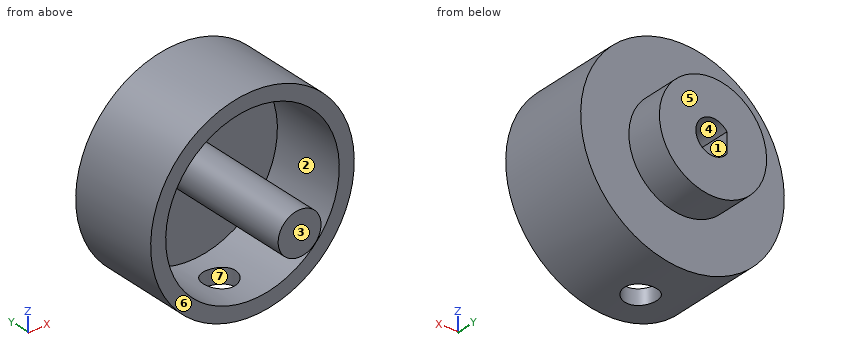
```python
from build123d import *

# Parameters (mm, degrees)
ESQUISSE1_R             = 4
BOSS_EXTRU_1_DEPTH      = 35
ESQUISSE2_R             = 3.2
ENL_V_MAT_EXTRU_1_DEPTH = 13
BOSS_EXTRU_2_START      = 13
BOSS_EXTRU_2_DEPTH      = 13
ESQUISSE5_R             = 10
ESQUISSE5_R_2           = 4
BOSS_EXTRU_3_DEPTH      = 7
SKETCH2_R               = 16.2
SKETCH2_R_2             = 4
BOSS_EXTRUDE4_DEPTH     = 3
SKETCH2_8_R             = 19
SKETCH2_8_R_2           = 16.2
BOSS_EXTRUDE5_DEPTH     = 17.2
SKETCH4_R               = 3
CUT_EXTRUDE1_DEPTH      = 10


with BuildPart() as part:
    # Esquisse1 → Boss.-Extru.1 (new body)
    with BuildSketch(Plane(origin=(0, 0, 0), x_dir=(1, 0, 0), z_dir=(0, 1, 0))):
        with Locations(Location((0, 0, 0), (0, 0, 270))):
            Circle(ESQUISSE1_R)
    extrude(amount=-BOSS_EXTRU_1_DEPTH)

    # Esquisse2 → Enl_v. mat.-Extru.1 (cut)
    with BuildSketch(Plane(origin=(0, 0, 0), x_dir=(1, 0, 0), z_dir=(0, 1, 0))):
        with Locations(Location((0, 0, 0), (0, 0, 270))):
            Circle(ESQUISSE2_R)
    extrude(amount=-ENL_V_MAT_EXTRU_1_DEPTH, mode=Mode.SUBTRACT)

    # Esquisse4 → Boss.-Extru.2 (add)
    with BuildSketch(Plane(origin=(0, -13, 0), x_dir=(1, 0, 0), z_dir=(0, 1, 0)).offset(BOSS_EXTRU_2_START)):
        with BuildLine():
            Line((-2.6, -1.865475811), (-2.6, 0))
            Line((-2.6, 0), (-2.6, 1.865475811))
            ThreePointArc((-2.6, 1.865475811), (-3.2, 0), (-2.6, -1.865475811))
        make_face()
    extrude(amount=-BOSS_EXTRU_2_DEPTH)

    # Esquisse5 → Boss.-Extru.3 (add)
    with BuildSketch(Plane(origin=(0, 0, 0), x_dir=(1, 0, 0), z_dir=(0, 1, 0))):
        with Locations(Location((0, 0, 0), (0, 0, 270))):
            Circle(ESQUISSE5_R)
        with Locations(Location((0, 0, 0), (0, 0, 270))):
            Circle(ESQUISSE5_R_2, mode=Mode.SUBTRACT)
    extrude(amount=-BOSS_EXTRU_3_DEPTH)

    # Sketch2 → Boss-Extrude4 (add)
    with BuildSketch(Plane.XZ.offset(7)):
        with Locations(Location((0, 0, 0), (0, 0, 270))):
            Circle(SKETCH2_R)
        with Locations(Location((0, 0, 0), (0, 0, 90))):
            Circle(SKETCH2_R_2, mode=Mode.SUBTRACT)
    extrude(amount=BOSS_EXTRUDE4_DEPTH)

    # Sketch2_8 → Boss-Extrude5 (add)
    with BuildSketch(Plane.XZ.offset(7)):
        with Locations(Location((0, 0, 0), (0, 0, 90))):
            Circle(SKETCH2_8_R)
        with Locations(Location((0, 0, 0), (0, 0, 90))):
            Circle(SKETCH2_8_R_2, mode=Mode.SUBTRACT)
    extrude(amount=BOSS_EXTRUDE5_DEPTH)

    # Sketch4 → Cut-Extrude1 (cut)
    with BuildSketch(Plane(origin=(0, 0, -19), x_dir=(-1, 0, 0), z_dir=(0, 0, -1))):
        with Locations((0, -16.6)):
            Circle(SKETCH4_R)
    extrude(amount=-CUT_EXTRUDE1_DEPTH, mode=Mode.SUBTRACT)


solid = part.part
```
Part model, mm, in its own coordinate system. Face numbers are marked on the shaded views. A direction names the side the tool comes from. Round coordinates to 2 decimals unless told otherwise and drop trailing zeros. Loops run counter-clockwise (first coordinate to the right, second up) from the corner with the lowest first, then second, coordinate; pieces in that order, holes last.
Item 1: Cut at A-A, the plane x = 0. Give the cut face in (y, z), then the cut area to 3 significant figures.
Item 2: Drill centre lines: line 1 (X direction, y = -18, z = 0); line 2 (Y direction, x = 0, z = -17.7); line 3 (X direction, y = -3, z = 0). Where is each one in solid material? Low to high.
Item 3: Drop flat-ended pins along their axis: P1, Ø8, axis at y = -28, z = 7.5, coming from the -X side; P2, Ø2, axis at x = 15, y = -10.5, coming from the +Z side; P3, Ø8, axis at y = -29, z = -1.5, coming from the -X side; P4, Ø6, axis at x = 0, z = 0, coming from the +Y side. Give the stop position or say it passes through.
Item 4: Cut at B-B, the plane y = -18. Give the cut face in (x, z).
Item 5: Cut at C-C, the plane z = -8.5. Give the cut face in (x, y), then the cut area to 3 significant figures.
Item 6: Mould opens along Y. For the marked faces 4, 5, 6 and 7 say: +Y half, -Y half, draft (parallel to the pull), parting line (faces both ways), or undercut.
Item 7: Cut at D-D, the plane x = 5. Give the cut face in (y, z), then the cut area to 3 significant figures.
Item 8: 3-axis set-ups, long thin cutter, end or side, ignore diameter. For the marked faces 1, 2 and 3: which of +Z, -Z, +X, -X, +Y, -Y reach the whole face in a straight line?
A:
1. outline: (-35, -4) - (-10, -4) - (-10, -16.2) - (-13.6, -16.2) - (-13.6, -19) - (-7, -19) - (-7, -10) - (0, -10) - (0, -3.2) - (-13, -3.2) - (-13, 3.2) - (0, 3.2) - (0, 10) - (-7, 10) - (-7, 19) - (-24.2, 19) - (-24.2, 16.2) - (-10, 16.2) - (-10, 4) - (-35, 4) - close; (-24.2, -19) - (-19.6, -19) - (-19.6, -16.2) - (-24.2, -16.2) - close
1. area: 434 mm2
2. line 1: x = -19 to -16.2, -4 to 4, 16.2 to 19
2. line 2: y = -24.2 to -19.6, -13.6 to -7
2. line 3: x = -10 to -2.6, 3.2 to 10
3. P1: stops at x = -17.94
3. P2: stops at z = 12.85
3. P3: stops at x = -4
3. P4: stops at y = 0
4. outline: circle Ø8 at (0, 0); (-2.65, -18.81) - (-2.65, -15.98) arc R16.2 cw (long way) to (2.65, -15.98) - (2.65, -18.81) arc R19 ccw (long way) to start
5. outline: (-16.99, -24.2) - (-13.79, -24.2) - (-13.79, -10) - (13.79, -10) - (13.79, -24.2) - (16.99, -24.2) - (16.99, -7) - (5.27, -7) - (5.27, 0) - (-5.27, 0) - (-5.27, -7) - (-16.99, -7) - close
5. area: 267 mm2
6. face 4: draft
6. face 5: +Y half
6. face 6: -Y half
6. face 7: undercut
7. outline: (-24.2, -18.33) - (-7, -18.33) - (-7, -8.66) - (0, -8.66) - (0, 8.66) - (-7, 8.66) - (-7, 18.33) - (-24.2, 18.33) - (-24.2, 15.41) - (-10, 15.41) - (-10, -15.41) - (-24.2, -15.41) - close
7. area: 314 mm2
8. face 1: +Y
8. face 2: -Y
8. face 3: +Z, -Z, +X, -X, -Y
